Verification items for the finished model (mm, model axes). Round coordinates to 2 decimals unless told otherwise and drop trailing zeros. Write each loop counter-clockwise with the first axis right and the second up, starting at its lowest first coordinate (ties: lowest second). Pieces come first, ordered by that corner, then holes. Notation, with made-up numbers: M 1,-18.5 L 14,-18.5 A11 ccw 14,-1.5 Z; hole C 33,73.25 d1. An arc over 180 degrees is marked long. One line per question, with ' | ' between items. Start each with the question number.
Q1. Thickness scan on line 1 along X through (y, z) = (-43, 3.95); line 2 along Y through (x, z) = (-34.75, 1.9); line 3 along X through (y, z) = (-18, 1.05). Record the ranges inside material, lowest first. Write a range as from..to.
Q2. Cross-section at C-C (y = -42.5). Record the boundary of the cut face in (x, z).
Q3. Release check for a two-part mould opening along X. For faces 1 (the face through (40.89, -1.63, 2.96)), 2 (the face through (14, -27, 6)), 3 (the face through (39.17, -8.44, 2.96)) record: released by +X, released by -X, zero draft, split by the parting line, or undercut.
Q4. Cross-section at A-A (z = 1.15). Record the boundary of the cut face in (x, y).
Q5. Gauge pin test, flat ends, axial feed: pin 1 (3 mm diameter, centred on y = -19, z = 1.5, fed in from -X) (3 decimals); pin 2 (10 mm diameter, centred on x = 35.5, y = -29, fed in from -Z). Record the tip position at first contact, or that the pin passes through.
Q6. Cross-section at D-D (y = -22.5). Record the boundary of the cut face in (x, z).
Q7. Cross-section at B-B (x = 0). Record the boundary of the cut face in (y, z).
from build123d import *
from build123d import SkipClean  # not in build123d's __all__

# Parameters (mm, degrees)
F0_R     = 6
F1_DEPTH = 6


with BuildPart() as f1:
    # F0 (on Top) → F1 (new body)
    with BuildSketch(Plane.XY):
        with BuildLine():
            Line((0, -16.5), (0, 0))
            Line((0, 0), (-35.4166666667, 0))
            ThreePointArc((-35.4166666667, 0), (-40.9636686289, -1.6794970566), (-44.6474358974, -6.1538461538))
            Line((-44.6474358974, -6.1538461538), (-59.2307692308, -41.1538461538))
            ThreePointArc((-59.2307692308, -41.1538461538), (-58.3205029434, -50.5470019623), (-50, -55))
            Line((-50, -55), (0, -55))
            Line((0, -55), (0, -45))
            ThreePointArc((0, -45), (-14.25, -30.75), (0, -16.5))
        make_face()
        with Locations((-47.25, -42.5)):
            Circle(F0_R, mode=Mode.SUBTRACT)
        with Locations((-34.75, -12.5)):
            Circle(F0_R, mode=Mode.SUBTRACT)
    extrude(amount=F1_DEPTH)

    # F2: F1 across plane


with BuildPart() as f1_1:
    add(f1.part, clean=False)
    with SkipClean():  # cleaning this boolean's faces spoils the solid; the shape is the same uncleaned
        add(f1.part.mirror(Plane.YZ), clean=False)


solid = f1_1.part
Determined:
1) line 1: x = -59.8..-53.23, -41.27..-7.28, 7.28..41.27, 53.23..59.8 | line 2: y = -55..-18.5, -6.5..0 | line 3: x = -49.58..-37.15, -32.35..-6.36, 6.36..32.35, 37.15..49.58
2) outline: M -59.68,0 L -53.25,0 L -53.25,6 L -59.68,6 Z; M -41.25,0 L -8.06,0 L -8.06,6 L -41.25,6 Z; M 8.06,0 L 41.25,0 L 41.25,6 L 8.06,6 Z; M 53.25,0 L 59.68,0 L 59.68,6 L 53.25,6 Z
3) face 1: released by +X | face 2: zero draft | face 3: undercut
4) outline: M -59.23,-41.15 A10 ccw -50,-55 L 50,-55 A10 ccw 59.23,-41.15 L 44.65,-6.15 A10 ccw 35.42,0 L -35.42,0 A10 ccw -44.65,-6.15 Z; hole C -47.25,-42.5 d12; hole C -34.75,-12.5 d12; hole C 0,-30.75 d28.5; hole C 34.75,-12.5 d12; hole C 47.25,-42.5 d12
5) pin 1: stops at x = -50.625 | pin 2: stops at z = 0
6) outline: M -51.46,0 L -11.62,0 L -11.62,6 L -51.46,6 Z; M 11.62,0 L 51.46,0 L 51.46,6 L 11.62,6 Z
7) outline: M -55,0 L -45,0 L -45,6 L -55,6 Z; M -16.5,0 L 0,0 L 0,6 L -16.5,6 Z
